Part model, mm, in its own coordinate system. A direction names the side the tool comes from. Give positions to 0.01 mm unless a question says otherwise; leave off trailing zeros. Order: outer loops, then holes, each group sorted by start corner. A loop starts at its lowest first (then second) coordinate and runs counter-clockwise, first axis right, second up. Notation, with made-up numbers: (19, 54) - (47, 54) arc R17 ccw to (47, 82) - close; hole circle Ø8 at (41.25, 12). An arc over 180 degrees is marked (long way). One line per item, written item: value.
```python
from build123d import *

# Parameters (mm, degrees)
SKETCH3_R               = 3.5
SKETCH3_R_2             = 2
BOSS_EXTRUDE1_DEPTH     = 2.5
SKETCH4_R               = 1.95
BOSS_EXTRUDE2_DEPTH     = 12.5
CUT_EXTRUDE1_DEPTH      = 10
CHAMFER1_SIZE           = 0.25
SKETCH6_R               = 2
CUT_EXTRUDE2_DEPTH      = 5
SKETCH7_R               = 1.75
BOSS_EXTRUDE3_DEPTH     = 5.2
CUT_EXTRUDE4_DEPTH      = 1
SKETCH9_R               = 1.25
CUT_EXTRUDE5_DEPTH      = 5
SKETCH11_W              = 0.2
SKETCH11_H              = 2
BOSS_EXTRUDE4_DEPTH     = 3
CUT_EXTRUDE6_START      = -20.2
CUT_EXTRUDE6_DEPTH      = 20.2
CUT_EXTRUDE7_DEPTH      = 62.520823074
CUT_EXTRUDE7_DEPTH_BACK = 62.520823074
SKETCH13_R              = 0.5


# Read off the part's stored shape, not the designer's step: Cut-Extrude6
with BuildPart() as part:
    # Sketch1 → Revolve1 (revolve)
    with BuildSketch(Plane.XY, mode=Mode.PRIVATE) as revolve1_sk:
        Polygon((-11.725797436, 0), (-11.725797436, 12), (19.274202564, 12), (19.274202564, 12.5), (24.274202564, 12.5), (24.274202564, 12.6), (38.274202564, 12.6), (38.274202564, 12.5), (43.274202564, 12.5), (43.274202564, 0), align=None)
    revolve(revolve1_sk.sketch.rotate(Axis((-11.725797436, 0, 0), (1, 0, 0)), 90), axis=Axis((-11.725797436, 0, 0), (1, 0, 0)))

    # Sketch3 → Boss-Extrude1 (add)
    with BuildSketch(Plane(origin=(43.274202564, 0, 0), x_dir=(0, 0, -1), z_dir=(1, 0, 0))):
        with Locations(Location((0, 0, 0), (0, 0, 180))):
            Circle(SKETCH3_R)
        Circle(SKETCH3_R_2, mode=Mode.SUBTRACT)
    extrude(amount=BOSS_EXTRUDE1_DEPTH)

    # Sketch4 → Boss-Extrude2 (add)
    with BuildSketch(Plane(origin=(43.274202564, 0, 0), x_dir=(0, 0, -1), z_dir=(1, 0, 0))):
        with Locations(Location((0, 0, 0), (0, 0, 180))):
            Circle(SKETCH4_R)
    extrude(amount=BOSS_EXTRUDE2_DEPTH)

    # Sketch5 → Cut-Extrude1 (cut)
    with BuildSketch(Plane(origin=(55.774202564, 0, 0), x_dir=(0, 0, -1), z_dir=(1, 0, 0))):
        with BuildLine():
            Line((0, 1.45), (1.563854219, 1.45))
            ThreePointArc((1.563854219, 1.45), (0.020575485, 2.299790468), (-1.52270325, 1.45))
            Line((-1.52270325, 1.45), (0, 1.45))
        make_face()
    extrude(amount=-CUT_EXTRUDE1_DEPTH, mode=Mode.SUBTRACT)

    # Chamfer1
    chamfer1_edges = [part.edges().sort_by_distance(p)[0] for p in [
        (19.274202564, 0, -12.5),
    ]]
    chamfer(chamfer1_edges, length=CHAMFER1_SIZE)

    # Sketch6 → Cut-Extrude2 (cut)
    with BuildSketch(Plane(origin=(43.274202564, 0, 0), x_dir=(0, 0, -1), z_dir=(1, 0, 0))):
        with Locations((10, 0)):
            Circle(SKETCH6_R)
        with Locations(Location((-10, 0, 0), (0, 0, 180))):
            Circle(SKETCH6_R)
    extrude(amount=-CUT_EXTRUDE2_DEPTH, mode=Mode.SUBTRACT)

    # Sketch7 → Boss-Extrude3 (add)
    with BuildSketch(Plane(origin=(38.274202564, 0, 0), x_dir=(0, 0, -1), z_dir=(1, 0, 0))):
        with Locations((10, 0)):
            Circle(SKETCH7_R)
        with Locations(Location((-10, 0, 0), (0, 0, 180))):
            Circle(SKETCH7_R)
    extrude(amount=BOSS_EXTRUDE3_DEPTH)

    # Sketch8 → Cut-Extrude4 (cut)
    with BuildSketch(Plane(origin=(43.474202564, 0, 0), x_dir=(0, 0, -1), z_dir=(1, 0, 0))):
        Polygon((8.594754122, -0.25), (8.594754122, 0.25), (9.75, 0.25), (9.75, 1.338286548), (10.25, 1.338286548), (10.25, 0.25), (11.405245878, 0.25), (11.405245878, -0.25), (10.25, -0.25), (10.25, -1.338286548), (9.75, -1.338286548), (9.75, -0.25), align=None)
        Polygon((-10.25, -0.25), (-11.405245878, -0.25), (-11.405245878, 0.25), (-10.25, 0.25), (-10.25, 1.338286548), (-9.75, 1.338286548), (-9.75, 0.25), (-8.594754122, 0.25), (-8.594754122, -0.25), (-9.75, -0.25), (-9.75, -1.338286548), (-10.25, -1.338286548), align=None)
    extrude(amount=-CUT_EXTRUDE4_DEPTH, mode=Mode.SUBTRACT)

    # Sketch9 → Cut-Extrude5 (cut)
    with BuildSketch(Plane(origin=(43.274202564, 0, 0), x_dir=(0, 0, -1), z_dir=(1, 0, 0))):
        with Locations((0, 8.5)):
            Circle(SKETCH9_R)
        with Locations(Location((0, -8.5, 0), (0, 0, 180))):
            Circle(SKETCH9_R)
    extrude(amount=-CUT_EXTRUDE5_DEPTH, mode=Mode.SUBTRACT)

    # Sketch11 → Boss-Extrude4 (add)
    with BuildSketch(Plane.ZY.offset(11.725797436)):
        with Locations((10, 0)):
            Rectangle(SKETCH11_W, SKETCH11_H)
        with Locations((-10, 0)):
            Rectangle(SKETCH11_W, SKETCH11_H)
    extrude(amount=BOSS_EXTRUDE4_DEPTH)

    # Cut-Extrude6 outline → Cut-Extrude6 (cut)
    with BuildSketch(Plane(origin=(0, 0, -10.1), x_dir=(-1, 0, 0), z_dir=(0, 0, -1)).offset(CUT_EXTRUDE6_START)):
        with BuildLine():
            ThreePointArc((13.765046185, 1), (14.446690478, 0.693369124), (14.725797436, 0))
            Line((14.725797436, 0), (14.725797436, 1))
            Line((14.725797436, 1), (13.765046185, 1))
        make_face()
        with BuildLine():
            ThreePointArc((14.725797436, 0), (14.446690478, -0.693369124), (13.765046185, -1))
            Line((13.765046185, -1), (14.725797436, -1))
            Line((14.725797436, -1), (14.725797436, 0))
        make_face()
    extrude(amount=CUT_EXTRUDE6_DEPTH, mode=Mode.SUBTRACT)

    # Sketch13 → Cut-Extrude7 (cut, two sides: drawn at the far end of the back side and taken through both)
    with BuildSketch(Plane(origin=(0, 0, -10.1), x_dir=(-1, 0, 0), z_dir=(0, 0, -1)).offset(-CUT_EXTRUDE7_DEPTH_BACK)):
        with Locations((13.724995738, 0)):
            Circle(SKETCH13_R)
    extrude(amount=CUT_EXTRUDE7_DEPTH + CUT_EXTRUDE7_DEPTH_BACK, mode=Mode.SUBTRACT)


solid = part.part
```
1) Drill centre lines: line 1 along Y through (x, z) = (39.7, 0); line 2 along X through (y, z) = (-3.5, 8.5); line 3 along Z through (x, y) = (7.5, 2.5). Where is each one in solid material? Low to high. Write a range as from..to.
Outcome:
line 1: y = -12.5..-9.75, -7.25..7.25, 9.75..12.5
line 2: x = -11.73..43.27
line 3: z = -11.74..11.74
2) Which spindle directions (+Z, -Z, +X, -X, +Y, -Y) get a long thin tool onto all of the face, cutting with end or side? Do faces 4 (the cylindrical face through (40.8, 1.2, 8.4)), 5 (the flat face through (-13, 0, -9.9)), 6 (the flat face through (43.474, -0.4, -10.4)), 7 (the cylindrical face through (31.372, 7.667, -9.999)). Say none if no direction does.
Outcome:
face 4: +X
face 5: -X, +Y, -Y
face 6: -Z, +X, +Y, -Y
face 7: +X, -X
3) Cut at C-C, the plane x = 20.5. Give the cut face in (y, z).
Outcome:
outline: circle Ø25 at (0, 0)
4) Mould opens along Z. For faces 1 (the cylindrical face through (40.81, -9.74, -0.16)), 2 (the flat face through (-13, 0, 10.1)), 3 (the cylindrical face through (21.932, -3.755, 11.923)) say: released by +Z, released by -Z, zero draft, split by the parting line, or undercut.
Outcome:
face 1: undercut
face 2: released by +Z
face 3: split by the parting line
5) Cut at B-B, the plane x = 48. Give the cut face in (y, z), then the cut area to 3 significant figures.
Outcome:
outline: (1.45, -1.3) - (1.45, 1.3) arc R1.95 ccw (long way) to start
area: 11.1 mm^2
6) Pin check, flat tips, straight feed: pin 1 (3 mm diameter, centred on x = 28, z = 8, fed in from -Y); pin 2 (1 mm diameter, centred on y = -7.5, z = 0.5, fed in from -X); pin 3 (6 mm diameter, centred on x = 20.5, y = -5.5, fed in from -Z). Stop position of each tip, or through.
Outcome:
pin 1: stops at y = -10.79
pin 2: stops at x = -11.73
pin 3: stops at z = -12.25
7) Cut at A-A, the plane x = 12.5. Give the cut face in (y, z), then the cut area to 3 significant figures.
Outcome:
outline: circle Ø24 at (0, 0)
area: 452 mm^2
